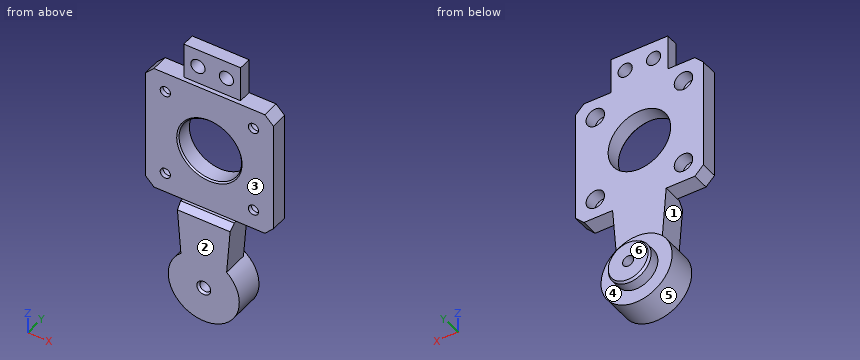
Solid Edge part; units mm, degrees
sketch "Sketch1" plane through (0, 0, 0) normal (1, 0, 0) x (0, 1, 0)
  line L0 (0, 1.95) -> (15, 1.95)
  line L1 (15, 1.95) -> (15, 7.5)
  line L2 (15, 7.5) -> (10.5, 7.5)
  line L3 (10.5, 7.5) -> (10.5, 12.5)
  line L4 (10.5, 12.5) -> (0, 12.5)
  line L5 (0, 12.5) -> (0, 1.95)
  dimension "D1" = 10.5
  dimension "D2" = 15
revolve "RevolvedProtrusion1" add sketch "Sketch1" angle 360 about axis through (0, -60, 0) along (0, 1, 0)
chamfer "Chamfer_1" distance 0.5 angle 60 1 edges at (0, 15, 7.5) measured on face at (-4.85, 15, 5.15)
sketch "Sketch2" plane through (0, 0, 0) normal (0, -1, 0) x (1, 0, 0)
  line L0 (-7.5, 2.5) -> (7.5, 2.5)
  line L1 (7.5, 2.5) -> (10, 35)
  line L2 (10, 85) -> (10, 35)
  line L3 (-10, 85) -> (10, 85)
  line L4 (-10, 35) -> (-10, 85)
  line L5 (-10, 35) -> (-7.5, 2.5)
  dimension "D1" = 10
  dimension "D2" = 7.5
extrude "ExtrudedProtrusion_1" add sketch "Sketch2" against normal blind 9
chamfer "Chamfer_2" distance 0.5 angle 60 1 edges at (0, 0, 1.95) measured on face at (-8.0833, 0, 2.775)
sketch "Sketch3" plane through (0, 9, 43.7496) normal (0, 1, 0) x (0, 0, -1)
  line L0 (-28.7504, 22.5) -> (-28.7504, -22.5)
  line L1 (-28.7504, -22.5) -> (16.2496, -22.5)
  line L2 (16.2496, -22.5) -> (16.2496, 22.5)
  line L3 (16.2496, 22.5) -> (-28.7504, 22.5)
  dimension "D1" = 28.7504
extrude "ExtrudedProtrusion_2" add sketch "Sketch3" against normal blind 9
sketch "Sketch4" plane through (0, 0, 36.25) normal (0, -1, 0) x (0, 0, 1)
  line L0 (-8.75, -22.5) -> (36.25, -22.5)
  line L1 (36.25, -22.5) -> (36.25, 22.5)
  line L2 (36.25, 22.5) -> (-8.75, 22.5)
  line L3 (-8.75, 22.5) -> (-8.75, -22.5)
extrude "ExtrudedCutout_1" cut sketch "Sketch4" against normal blind 3
hole "Hole_1" at (0, 3, 50) direction (0, 1, 0) diameter 8 end up to next
hole "Hole_2" at (15.5, 9, 65.5) direction (0, -1, 0) diameter 3.6 end up to next counterbore diameter 6.5 counterbore depth 4.5
hole "Hole1" at (-15.5, 9, 65.5) direction (0, -1, 0) diameter 3.6 end up to next counterbore diameter 6.5 counterbore depth 4.5
hole "Hole2" at (-15.5, 9, 34.5) direction (0, -1, 0) diameter 3.6 end up to next counterbore diameter 6.5 counterbore depth 4.5
hole "Hole3" at (15.5, 9, 34.5) direction (0, -1, 0) diameter 3.6 end up to next counterbore diameter 6.5 counterbore depth 4.5
sketch "Sketch5" plane through (0, 4.5, 85) normal (0, 0, 1) x (0, 1, 0)
  line L0 (-4.5, 10) -> (0, 10)
  line L1 (0, 10) -> (0, -10)
  line L2 (0, -10) -> (-4.5, -10)
  line L3 (-4.5, -10) -> (-4.5, 10)
extrude "ExtrudedCutout_2" cut sketch "Sketch5" against normal blind 12.5
hole "Hole_6" at (5, 9, 78.75) direction (0, -1, 0) diameter 5 end up to next
hole "Hole4" at (-5, 9, 78.75) direction (0, -1, 0) diameter 5 end up to next
chamfer "Chamfer_3" distance 3 angle 45 4 edges at (22.5, 6, 27.5) (22.5, 6, 72.5) (-22.5, 6, 72.5) (-22.5, 6, 27.5)
chamfer "Chamfer_4" distance 2 angle 45 1 edges at (0, 0, 27.5)
hole "Hole_8" at (0, 3, 50) direction (0, 1, 0) diameter 22 depth 50.8
chamfer "Chamfer_5" distance 0.5 angle 45 1 edges at (0, 3, 61)
properties material "Polyethylene, low density"
Model file for the job. Use its own axes, mm. Face numbers are marked on the shaded views. A direction names the side the tool comes from. Round coordinates to 2 decimals unless told otherwise and drop trailing zeros. Order: outer loops, then holes, each group sorted by start corner. A loop starts at its lowest first (then second) coordinate and runs counter-clockwise, first axis right, second up.
(1) Pull direction Z, two halves, no side cores. Call the marked faces 5 and 6: released by +Z, released by -Z, zero draft, split by the parting line, or undercut.
(2) 3-axis set-ups, long thin cutter, end or side, ignore diameter. For the marked faces 1, 2, 3 and 4: which of +Z, -Z, +X, -X, +Y, -Y reach the whole face in a straight line?
(3) Band-saw the part on A-A (z = 50). List the corners of the cut face in (x, y).
(4) Band-saw the part on C-C (x = 0). Give the number of separate pieces and of enclosed holes in the cut face, then the cut area to 3 significant figures.
(5) Drill centre lines: line 1 (X direction, y = 3.75, z = 65.5); line 2 (Z direction, x = -15.5, y = 6.15); line 3 (Z direction, x = 15.5, y = 4.2). Where is each one in solid material? Low to high.
(6) Pin check, flat tips, straight feed: pin 1 (4 mm diameter, centred on x = 5.5, y = 6.5, fed in from -Z); pin 2 (5 mm diameter, centred on y = 7, z = 4.5, fed in from +X); pin 3 (12 mm diameter, centred on x = 5, z = 63, fed in from +Y). Stop position of each tip, or through.
(7) Band-saw the part on B-B (z = 34.5). List the corners of the cut face in (x, y), then the cut area to 3 significant figures.
Verdict:
1. face 5: undercut
1. face 6: zero draft
2. face 1: -X, +Y, -Y
2. face 2: +Z, -Z, +X, -X, -Y
2. face 3: +Z, +X, -X, -Y
2. face 4: +Y
3. outline: (-22.5, 3) - (-11.5, 3) - (-11, 3.5) - (-11, 9) - (-22.5, 9) - close; (11, 3.5) - (11.5, 3) - (22.5, 3) - (22.5, 9) - (11, 9) - close
4. separate pieces: 3
4. enclosed holes: 0
4. area: 598 mm2
5. line 1: x = -22.5 to -17.3, -13.7 to 13.7, 17.3 to 22.5
5. line 2: z = 27.5 to 31.25, 37.75 to 62.25, 68.75 to 72.5
5. line 3: z = 27.5 to 32.7, 36.3 to 63.7, 67.3 to 72.5
6. pin 1: stops at z = -12
6. pin 2: stops at x = 12.34
6. pin 3: stops at y = 9
7. outline: (-22.5, 3) - (-17.3, 3) - (-17.3, 4.5) - (-18.75, 4.5) - (-18.75, 9) - (-22.5, 9) - close; (-13.7, 3) - (13.7, 3) - (13.7, 4.5) - (12.25, 4.5) - (12.25, 9) - (-12.25, 9) - (-12.25, 4.5) - (-13.7, 4.5) - close; (17.3, 3) - (22.5, 3) - (22.5, 9) - (18.75, 9) - (18.75, 4.5) - (17.3, 4.5) - close
7. area: 201 mm2
